The listing builds one solid part. Answer for the finished solid, in the listing's coordinates (mm). A direction names the side the tool comes from. Round coordinates to 2 decimals unless told otherwise and drop trailing zeros. Write each loop counter-clockwise with the first axis right and the second up, starting at its lowest first coordinate (ties: lowest second). Pieces come first, ordered by that corner, then holes. Notation, with made-up numbers: (12, 63) - (71, 63) arc R30 ccw to (71, 101) - close; hole circle Ø11 at (32.5, 14.5). An arc over 180 degrees is marked (long way). Answer in a Markdown table with one row per item.
from build123d import *

# Parameters (mm, degrees)
F0_W        = 6.1
F0_H        = 3
F0_W_2      = 27.8
F1_DEPTH    = 40
F2_R        = 1
F3_T1_DEPTH = 168.4279953904
F4_DEPTH    = 22


# Not quite as in the source:
# - a fillet or chamfer that OpenCascade refuses, or shapes differently, is made with other operations: its cross-section is extruded or revolved along the edge and cut away or added


with BuildPart() as f1:
    # F0 (on Top) → F1 (new body)
    with BuildSketch(Plane.XY):
        with Locations((3.05, 6.91)):
            Rectangle(F0_W, F0_H)
        with Locations((-3.05, 6.91)):
            Rectangle(F0_W, F0_H)
        with BuildLine():
            Line((6.1, -1.59), (6.1, 5.41))
            Line((6.1, 5.41), (0, 5.41))
            Line((0, 5.41), (0, 2.15))
            ThreePointArc((0, 2.15), (1.5202795796, 1.5202795796), (2.15, 0))
            ThreePointArc((2.15, 0), (1.5202795796, -1.5202795796), (0, -2.15))
            Line((0, -2.15), (0, -6.09))
            Line((0, -6.09), (2.25, -6.09))
            ThreePointArc((2.25, -6.09), (4.7073896383, -4.2954889128), (6.1, -1.59))
        make_face()
        with Locations((20, 6.91)):
            Rectangle(F0_W_2, F0_H)
        with BuildLine():
            Line((33.9, 5.41), (6.1, 5.41))
            Line((6.1, 5.41), (6.1, -1.59))
            ThreePointArc((6.1, -1.59), (4.7073896383, -4.2954889128), (2.25, -6.09))
            Line((2.25, -6.09), (33.9, -6.09))
            Line((33.9, -6.09), (33.9, 5.41))
        make_face()
        with BuildLine():
            Line((0, 2.15), (0, 5.41))
            Line((0, 5.41), (-6.1, 5.41))
            Line((-6.1, 5.41), (-6.1, -1.59))
            ThreePointArc((-6.1, -1.59), (-4.7073896383, -4.2954889128), (-2.25, -6.09))
            Line((-2.25, -6.09), (0, -6.09))
            Line((0, -6.09), (0, -2.15))
            ThreePointArc((0, -2.15), (-2.15, 0), (0, 2.15))
        make_face()
    extrude(amount=F1_DEPTH)

    # F2
    f2_edges = [f1.edges().sort_by_distance(p)[0] for p in [
        (-2.25, -6.09, 20),
    ]]
    fillet(f2_edges, radius=F2_R)

    # F3: fillet of radius 30 on 1 edges, made by hand

    # F3_s2 → F3_t1 (cut)
    with BuildSketch(Plane.XY.offset(-64.2139976952)):
        with BuildLine():
            ThreePointArc((8.2144009219, -6.09), (22.9622821257, -2.2147009552), (33.9, 8.41))
            Line((33.9, 8.41), (33.9, -6.09))
            Line((33.9, -6.09), (8.2144009219, -6.09))
        make_face()
    extrude(amount=F3_T1_DEPTH, mode=Mode.SUBTRACT)

    # F0 (on Top) → F4 (cut)
    with BuildSketch(Plane.XY):
        with Locations((-3.05, 6.91)):
            Rectangle(F0_W, F0_H)
        with Locations((3.05, 6.91)):
            Rectangle(F0_W, F0_H)
        with Locations((20, 6.91)):
            Rectangle(F0_W_2, F0_H)
    extrude(amount=F4_DEPTH, mode=Mode.SUBTRACT)


solid = f1.part
(1) Section D-D (x = 13) is taken. Give the vertices of the cut face in (y, z), and give its area (3 significant figures).
Checked values:
| item | result |
|---|---|
| outline | (-5.71, 0) - (5.41, 0) - (5.41, 22) - (8.41, 22) - (8.41, 40) - (-5.71, 40) - close |
| area | 499 mm2 |
(2) Section A-A (z = 19) is taken. Give the vertices of the cut face in (x, y).
Checked values:
| item | result |
|---|---|
| outline | (-6.1, -1.59) arc R6.61 ccw to (-2.46, -6) arc R1 ccw to (-2.04, -6.09) - (8.21, -6.09) arc R30 ccw to (31.83, 5.41) - (-6.1, 5.41) - close; hole circle Ø4.3 at (0, 0) |
(3) Section C-C (z = 35) is taken. Give the vertices of the cut face in (x, y).
Checked values:
| item | result |
|---|---|
| outline | (-6.1, -1.59) arc R6.61 ccw to (-2.46, -6) arc R1 ccw to (-2.04, -6.09) - (8.21, -6.09) arc R30 ccw to (33.9, 8.41) - (-6.1, 8.41) - close; hole circle Ø4.3 at (0, 0) |
(4) Flat-ended cylindrical pins translate along their axes: pin 1 (0.9 mm diameter, centred on x = 7.5, y = 6, fed in from -Z); pin 2 (1 mm diameter, centred on x = 27.5, z = 9, fed in from -Y); pin 3 (5 mm diameter, centred on x = 10.5, y = -2, fed in from -Z); pin 4 (11 mm diameter, centred on x = 5.5, z = 7, fed in from +Y). Find the tip coordinate at first contact, or state that the pin passes through.
Checked values:
| item | result |
|---|---|
| pin 1 | stops at z = 22 |
| pin 2 | stops at y = 0.52 |
| pin 3 | stops at z = 0 |
| pin 4 | stops at y = 5.41 |
(5) Section B-B (x = 6) is taken. Give the vertices of the cut face in (y, z).
Checked values:
| item | result |
|---|---|
| outline | (-6.09, 0) - (5.41, 0) - (5.41, 22) - (8.41, 22) - (8.41, 40) - (-6.09, 40) - close |
(6) For faces 1 (the flat face through (8, 1, 0)), 2 (the flat face through (13, 5.41, 11)), determine the directions among +Z, -Z, +X, -X, +Y, -Y from which every point of the face is accessible in a straight line to the end or side of a thin tool.
Checked values:
| item | result |
|---|---|
| face 1 | -Z, +X, -X, +Y, -Y |
| face 2 | -Z, +X, -X, +Y |
(7) Find the intervals of material crossed by line 1 (Y direction, x = 24, z = 33); line 2 (Y direction, x = 4, z = 7.5); line 3 (X direction, y = 1.25, z = 20), in increasing order.
Checked values:
| item | result |
|---|---|
| line 1 | y = -1.6 to 8.41 |
| line 2 | y = -6.09 to 5.41 |
| line 3 | x = -6.1 to -1.75, 1.75 to 27.87 |
